Autodesk Inventor part; units mm, degrees
ref_plane "YZ Plane" through (0, 0, 0) normal (1, 0, 0) x (0, 1, 0)
ref_plane "XZ Plane" through (0, 0, 0) normal (0, 1, 0) x (-1, 0, 0)
ref_plane "XY Plane" through (0, 0, 0) normal (0, 0, 1) x (1, 0, 0)
sketch "Sketch1" plane through (0, 0, 0) normal (0, 1, 0) x (-1, 0, 0)
  line L0 (0, 0) -> (12, 0)
  line L1 (12, 0) -> (12, -15)
  line L2 (12, -15) -> (0, -15)
  line L3 (0, -15) -> (0, 0)
  dimension "d0" = 12
  dimension "d1" = 15
extrude "Extrusion1" add sketch "Sketch1" along normal blind 12
sketch "Sketch4" plane through (0, 0, 0) normal (0, -1, 0) x (1, 0, 0)
  line L0 (0, -15) -> (-12, -15)
  arc A0 (-12, -15) -> (0, -15) centre (-6, -15) ccw
  point P0 (0, 0)
  point P1 (-6, -15)
extrude "Extrusion2" add sketch "Sketch4" against normal up to surface (12 mm away)
sketch "Sketch5" plane through (0, 0, 0) normal (1, 0, 0) x (0, 0, -1)
  line L0 (3, 9.5) -> (21, 9.5)
  line L1 (21, 9.5) -> (21, 2.5)
  line L2 (21, 2.5) -> (3, 2.5)
  line L3 (3, 2.5) -> (3, 9.5)
  line L4 (15, 12) -> (15, 12)
  line L5 (15, 0) -> (15, 12)
  line L6 (15, 0) -> (15, 0)
  line L7 (15, 0) -> (15, 12)
  line L8 (21, 0) -> (21, 12)
  line L9 (0, 0) -> (0, 12)
  point P0 (21, 6)
  point P1 (3, 6)
  point P2 (0, 6)
  dimension "d8" = 18
  dimension "d9" = 7
extrude "Extrusion3" cut sketch "Sketch5" against normal up to surface (12 mm away)
sketch "Sketch6" plane through (0, 12, 0) normal (0, 1, 0) x (1, 0, 0)
  arc A0 (0, 15) -> (-12, 15) centre (-6, 15) ccw
  point P0 (0, 0)
hole "Hole1" at (-6, 12, -15) direction (0, -1, 0) diameter 5 depth 12
sketch "Sketch7" plane through (-12, 0, 0) normal (0, 0, 1) x (1, 0, 0)
  line L0 (10.5, 1.5) -> (1.5, 1.5)
  line L1 (1.5, 1.5) -> (1.5, 10.5)
  line L2 (1.5, 10.5) -> (10.5, 10.5)
  line L3 (10.5, 10.5) -> (10.5, 1.5)
  line L4 (0, 0) -> (0, 12)
  line L5 (0, 0) -> (12, 0)
  point P0 (1.5, 6)
  point P1 (0, 6)
  point P2 (6, 1.5)
  point P3 (6, 0)
  dimension "d19" = 9
  dimension "d20" = 9
extrude "Extrusion4" add sketch "Sketch7" along normal blind 5
fillet "Fillet1" radius 2 4 edges at (-6, 1.5, 0) (-10.5, 6, 0) (-6, 10.5, 0) (-1.5, 6, 0)
sketch "Sketch8" plane through (-12, 0, 5) normal (0, 0, 1) x (1, 0, 0)
  line L0 (10.5, 1.5) -> (10.5, 10.5)
  line L1 (1.5, 1.5) -> (10.5, 1.5)
  point P0 (12, 0)
  point P1 (6, 6)
  point P2 (10.5, 6)
  point P3 (6, 1.5)
hole "Hole2" at (-6, 6, 5) direction (0, 0, -1) diameter 4.134 depth 8
properties part number "2063"
The listing builds one solid part. Answer for the finished solid, in the listing's coordinates (mm). A direction names the side the tool comes from. Round coordinates to 2 decimals unless told otherwise and drop trailing zeros. Order: outer loops, then holes, each group sorted by start corner. A loop starts at its lowest first (then second) coordinate and runs counter-clockwise, first axis right, second up. Notation, with made-up numbers: (-6, 39.25) -> (20, 39.25) arc R23 ccw to (20, 74.25) -> close; hole circle Ø1 at (42.5, 34). An arc over 180 degrees is marked (long way). Write each question's results on one line, items separated by ' | '. Start each with the question number.
Q1. Each of these flat-tipped pins is pushed along its axis until it touches: pin 1 (5 mm diameter, centred on x = -10.5, y = 1.5, fed in from -Z); pin 2 (1 mm diameter, centred on x = -3, y = 4, fed in from -Z); pin 3 (0.9 mm diameter, centred on y = 7, z = 3, fed in from +X). Where does it stop, or does it pass through?
Q2. Straight lines are drawn through the part: probe 1 along Y at (x, z) = (-8, -5.5); probe 2 along Z at (x, y) = (-6, 1.85); probe 3 along Y at (x, z) = (-6, -0.75). For each, find the intervals that lie inside material, in ascending order. Write a range as from..to.
Q3. Which of the six approach directions +Z, -Z, +X, -X, +Y, -Y give full straight-line access (tool end or side, diameter ignored) to faces 1 (the flat face through (-10.5, 6, 3)), 2 (the flat face through (-6, 2.5, -12)), 3 (the flat face through (-1.5, 6, 3)), 4 (the flat face through (-6, 10.5, 3)), 5 (the flat face through (-6, 1.5, 3))?
Q4. Find section C-C (y = 5). Determine the outline of the cut face in (x, z).
Q5. Find section B-B (x = -6). Determine the outline of the cut face in (y, z).
Q6. Find section D-D (y = 9.75). Determine the outline of the cut face in (x, z), then the cut area to 3 significant figures.
Q7. The mould has two halves that part along Y. Classify faces 6 (the cylindrical face through (-5.92, 1.07, 0.7)), 7 (the flat face through (-5, 4, -3)), 8 (the flat face through (-12, 6, -2)): pulls with the +Y half, pulls with the -Y half, needs draft (parallel to the pull), parting line crosses it, or undercut.
Q8. Find section A-A (z = -8). Determine the outline of the cut face in (x, y).
Worked answers:
1) pin 1: stops at z = -20.66 | pin 2: stops at z = -3 | pin 3: stops at x = -1.5
2) probe 1: y = 0..2.5, 9.5..12 | probe 2: z = -21..-17.5, -12.5..5 | probe 3: y = 0..3.93, 8.07..12
3) face 1: +Z, -X, +Y, -Y | face 2: -Z, +X, -X | face 3: +Z, +X, +Y, -Y | face 4: +Z, +X, -X, +Y | face 5: +Z, +X, -X, -Y
4) outline: (-12, -3) -> (-7.81, -3) -> (-7.81, 5) -> (-10.5, 5) -> (-10.5, 1.94) arc R2 cw to (-12, 0) -> close; (-4.19, -3) -> (0, -3) -> (0, 0) arc R2 cw to (-1.5, 1.94) -> (-1.5, 5) -> (-4.19, 5) -> close
5) outline: (0, -21) -> (2.5, -21) -> (2.5, -17.5) -> (0, -17.5) -> close; (0, -12.5) -> (2.5, -12.5) -> (2.5, -3) -> (3.93, -3) -> (3.93, 5) -> (1.5, 5) -> (1.5, 1.94) arc R2 cw to (0, 0) -> close; (8.07, -3) -> (9.5, -3) -> (9.5, -12.5) -> (12, -12.5) -> (12, 0) arc R2 cw to (10.5, 1.94) -> (10.5, 5) -> (8.07, 5) -> close; (9.5, -21) -> (12, -21) -> (12, -17.5) -> (9.5, -17.5) -> close
6) outline: (-12, -15) arc R6 ccw to (0, -15) -> (0, 0) arc R2 cw to (-1.5, 1.94) -> (-1.5, 5) -> (-10.5, 5) -> (-10.5, 1.94) arc R2 cw to (-12, 0) -> close; hole circle Ø5 at (-6, -15) | area: 263 mm2
7) face 6: pulls with the -Y half | face 7: undercut | face 8: needs draft
8) outline: (-12, 0) -> (0, 0) -> (0, 2.5) -> (-12, 2.5) -> close; (-12, 9.5) -> (0, 9.5) -> (0, 12) -> (-12, 12) -> close
